from build123d import *

# Parameters (mm, degrees)
F1_DEPTH = 101.6
F2_R     = 13.97
F3_DEPTH = 5.08
F4_R     = 13.97
F5_DEPTH = 5.08
F6_R     = 13.97
F7_DEPTH = 5.08


with BuildPart() as f1:
    # F0 (on Top) → F1 (new body)
    with BuildSketch(Plane.XY):
        Polygon((-50.1161357684, 10.6036934298), (-15.875, -48.7036934298), (15.875, -48.7036934298), (50.1161357684, 10.6036934298), (34.2411357684, 38.1), (-34.2411357684, 38.1), align=None)
    extrude(amount=F1_DEPTH)

    # F2 (on face) → F3 (join)
    with BuildSketch(Plane(origin=(-32.9955678842, -19.05, 0), x_dir=(0.5, -0.8660254038, 0), z_dir=(-0.8660254038, -0.5, 0))):
        with Locations((0, 76.2)):
            Circle(F2_R)
        with Locations((0, 25.4)):
            Circle(F2_R)
    extrude(amount=F3_DEPTH)

    # F4 (on face) → F5 (join)
    with BuildSketch(Plane(origin=(0, 38.1, 0), x_dir=(-1, 0, 0), z_dir=(0, 1, 0))):
        with Locations((0, 76.2)):
            Circle(F4_R)
        with Locations((0, 25.4)):
            Circle(F4_R)
    extrude(amount=F5_DEPTH)

    # F6 (on face) → F7 (join)
    with BuildSketch(Plane(origin=(32.9955678842, -19.05, 0), x_dir=(0.5, 0.8660254038, 0), z_dir=(0.8660254038, -0.5, 0))):
        with Locations((0, 76.2)):
            Circle(F6_R)
        with Locations((0, 25.4)):
            Circle(F6_R)
    extrude(amount=F7_DEPTH)


solid = f1.part
The model under review builds one solid part; all positions refer to its coordinate system, in mm. A direction names the side the tool comes from. Round coordinates to 2 decimals unless told otherwise and drop trailing zeros. Write each loop counter-clockwise with the first axis right and the second up, starting at its lowest first coordinate (ties: lowest second). Pieces come first, ordered by that corner, then holes. Notation, with made-up numbers: (72, -4) - (95, -4) arc R19 cw to (95, 28) - close; hole circle Ø9 at (66, 10.5). An arc over 180 degrees is marked (long way). One line per item, written item: value. Start each with the question number.
1. Clearance check with flat-ended pins moving along their axes: P1, Ø1, axis at x = -23, z = 37, coming from the -Y side; P2, Ø8, axis at x = -39.5, z = 77, coming from the -Y side; P3, Ø8, axis at x = -38.5, z = 83.5, coming from the +Y side. State where each tip first meets the part, or that it passes through.
2. Consider section A-A on x = 0. Write out the cut boundary in (y, z), and give its area (3 significant figures).
3. Consider section B-B on z = 6. Write out the cut boundary in (x, y) (3 decimals).
4. To check wall thickness, follow L1, parallel to X at y = -31, z = 84.5; L2, parallel to Y at x = -10.5, z = 13.5; L3, parallel to Y at x = -39.5, z = 87. State the ranges of each line that lie inside material, in increasing order. Write a range as from..to.
5. Consider section D-D on z = 76.2. Write out the cut boundary in (x, y) (3 decimals), and give its area (3 significant figures).
6. Consider section C-C on y = -3. Write out the cut boundary in (x, z).
7. Machinability: for faces 1 (the face through (0, 38.1, 50)), 2 (the face through (-1, 5, 0)), which of the approach directions +Z, -Z, +X, -X, +Y, -Y give a long, thin tool a straight path to every point of the face, cutting with its end or side? Answer none if there is none.
8. The part is to be moulded in two halves that separate along Y. For faces 3 (the face through (42.29, 24.16, 50.09)), 4 (the face through (38.92, -13.8, 87.98)), 5 (the face through (0, -48.704, 50)), say which applies: released by +Y, released by -Y, zero draft, split by the parting line, or undercut.
Checks:
1. P1: stops at y = -37.23
1. P2: stops at y = -24.87
1. P3: stops at y = 37.65
2. outline: (-48.7, 0) - (38.1, 0) - (38.1, 11.43) - (43.18, 11.43) - (43.18, 39.37) - (38.1, 39.37) - (38.1, 62.23) - (43.18, 62.23) - (43.18, 90.17) - (38.1, 90.17) - (38.1, 101.6) - (-48.7, 101.6) - close
2. area: 9,100 mm^2
3. outline: (-50.116, 10.604) - (-15.875, -48.704) - (15.875, -48.704) - (50.116, 10.604) - (34.241, 38.1) - (-34.241, 38.1) - close
4. L1: x = -31.96..-31.22, -26.1..26.1, 31.22..31.96
4. L2: y = -48.7..38.1
4. L3: y = -17.94..-12.57, -7.78..28.99
5. outline: (-50.116, 10.604) - (-39.981, -6.952) - (-44.38, -9.492) - (-30.41, -33.688) - (-26.011, -31.148) - (-15.875, -48.704) - (15.875, -48.704) - (26.011, -31.148) - (30.41, -33.688) - (44.38, -9.492) - (39.981, -6.952) - (50.116, 10.604) - (34.241, 38.1) - (13.97, 38.1) - (13.97, 43.18) - (-13.97, 43.18) - (-13.97, 38.1) - (-34.241, 38.1) - close
5. area: 6,660 mm^2
6. outline: (-42.26, 0) - (42.26, 0) - (42.26, 101.6) - (-42.26, 101.6) - close
7. face 1: +Y
7. face 2: -Z, +X, -X, +Y, -Y
8. face 3: released by +Y
8. face 4: undercut
8. face 5: released by -Y
